Design review of the part shown in the three views and the two pictorial views. Dimensions are in mm from the part's minimum x, y and z. Give positions to 0.01 mm unless a question says otherwise; leave off trailing zeros. Loops run counter-clockwise (first coordinate to the right, second up) from the corner with the lowest first, then second, coordinate; pieces in that order, holes last.
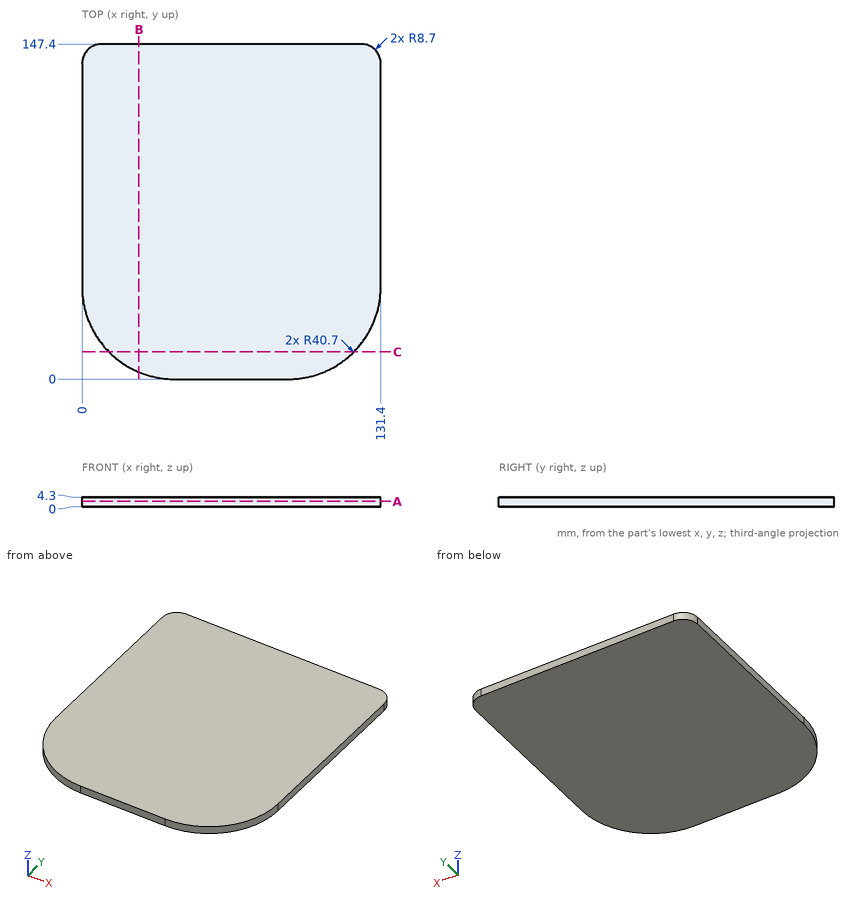
Q1. Consider section C-C on y = 12. Give the boundary of the cut face in (x, z).
Answers:
outline: (11.84, 0) - (119.56, 0) - (119.56, 4.3) - (11.84, 4.3) - close
Q2. Consider section B-B on x = 25. Give the boundary of the cut face in (y, z).
Answers:
outline: (3.15, 0) - (147.4, 0) - (147.4, 4.3) - (3.15, 4.3) - close
Q3. For pin 1 Ø2 at (y, z) = (47.5, 2) entering from -X, flat-tipped, find the tip position at first contact; note if it passes through.
Answers:
pin 1: stops at x = 0
Q4. Consider section A-A on z = 2.5. Give the boundary of the cut face in (x, y).
Answers:
outline: (0, 40.7) arc R40.7 ccw to (40.7, 0) - (90.7, 0) arc R40.7 ccw to (131.4, 40.7) - (131.4, 138.7) arc R8.7 ccw to (122.7, 147.4) - (8.7, 147.4) arc R8.7 ccw to (0, 138.7) - close
Q5. For probe 1 along Y at (x, z) = (126.5, 0.3); probe 2 along Y at (x, z) = (110, 2.55); probe 3 along X at (y, z) = (31.5, 3.1), list the stretches that pass through material, from the lowest coordinate up.
Answers:
probe 1: y = 21.34 to 146.53
probe 2: y = 4.87 to 147.4
probe 3: x = 1.05 to 130.35
